```python
from build123d import *

# Parameters (mm, degrees)
SKETCH1_W                       = 1.5
SKETCH1_H                       = 25
BOSS_EXTRUDE1_DEPTH             = 73
BOSS_EXTRUDE1_DEPTH_BACK        = 73
FILLET1_R                       = 1
BOSS_EXTRUDE2_REACH             = 2.75
SKETCH10_W                      = 20
SKETCH10_H                      = 25
BOSS_EXTRUDE2_DIRECTION_2_REACH = 2.75
SKETCH16_W                      = 40.5
SKETCH16_H                      = 3
CUT_EXTRUDE2_DEPTH              = 10
SKETCH21_W                      = 65
SKETCH21_H                      = 47
BOSS_EXTRUDE4_DEPTH             = 1.5
FILLET4_R                       = 1.5
SKETCH17_W                      = 22.5
SKETCH17_H                      = 25
BOSS_EXTRUDE3_DEPTH             = 1.5
M2_CLEARANCE_HOLE4_D            = 2.4
M2_CLEARANCE_HOLE4_DEPTH        = 1.5
SKETCH22_OUTSIDE_W              = 183.058
SKETCH22_OUTSIDE_H              = 134.058
SKETCH22_OUTSIDE_W_2            = 125
SKETCH22_OUTSIDE_H_2            = 119
CUT_EXTRUDE4_DEPTH              = 10
M2_CLEARANCE_HOLE5_D            = 2.4
M2_CLEARANCE_HOLE5_DEPTH        = 11.5
SKETCH25_W                      = 65
SKETCH25_H                      = 2.5
SKETCH25_H_2                    = 0.5
BOSS_EXTRUDE5_DEPTH             = 1.5
M2_5_CLEARANCE_HOLE1_D          = 2.9
M2_5_CLEARANCE_HOLE1_DEPTH      = 11.5
SKETCH29_W                      = 7.5
SKETCH29_H                      = 30.5
SKETCH29_H_2                    = 50.5
CUT_EXTRUDE5_DEPTH              = 10
SKETCH31_W                      = 15
SKETCH31_H                      = 20.5
SKETCH31_H_2                    = 40.5
CUT_EXTRUDE7_DEPTH              = 10
FILLET5_R                       = 3
CHAMFER1_SIZE                   = 1.2
CHAMFER2_SIZE                   = 3
M2_5_CLEARANCE_HOLE2_D          = 2.9
M2_5_CLEARANCE_HOLE2_DEPTH      = 10


with BuildPart() as part:
    # Sketch1 → Boss-Extrude1 (new body, two sides)
    with BuildSketch(Plane.XY) as boss_extrude1_sk:
        Rectangle(SKETCH1_W, SKETCH1_H)
    extrude(amount=BOSS_EXTRUDE1_DEPTH)
    extrude(boss_extrude1_sk.sketch, amount=-BOSS_EXTRUDE1_DEPTH_BACK)

    # Fillet1
    fillet1_edges = [part.edges().sort_by_distance(p)[0] for p in [
        (0, -12.5, 73),
        (0, 12.5, -73),
        (0, 12.5, 73),
        (0, -12.5, -73),
    ]]
    fillet(fillet1_edges, radius=FILLET1_R)

    # Boss-Extrude2: up to this face of the body (flat: up to its plane)
    boss_extrude2_end = Plane(part.part.faces().sort_by_distance((0.75, 0, 0))[0])
    # Sketch10 → Boss-Extrude2 (add, up to the picked face)
    with BuildSketch(Plane(origin=(0, 0, 0), x_dir=(0, 0, -1), z_dir=(1, 0, 0)), mode=Mode.PRIVATE) as boss_extrude2_sk1:
        with Locations((0, 25)):
            Rectangle(SKETCH10_W, SKETCH10_H)
    boss_extrude2_tool1 = split(extrude(boss_extrude2_sk1.sketch, amount=BOSS_EXTRUDE2_REACH, mode=Mode.PRIVATE), bisect_by=boss_extrude2_end, keep=Keep.BOTH, mode=Mode.PRIVATE)
    add(boss_extrude2_tool1.solids().sort_by_distance((0, 25, 0))[0])

    # Boss-Extrude2 direction 2: up to this face of the body (flat: up to its plane)
    boss_extrude2_direction_2_end = Plane(part.part.faces().sort_by_distance((-0.75, 0, 0))[0])
    # Sketch10 → Boss-Extrude2 direction 2 (add, up to the picked face)
    with BuildSketch(Plane(origin=(0, 0, 0), x_dir=(0, 0, -1), z_dir=(1, 0, 0)), mode=Mode.PRIVATE) as boss_extrude2_direction_2_sk1:
        with Locations((0, 25)):
            Rectangle(SKETCH10_W, SKETCH10_H)
    boss_extrude2_direction_2_tool1 = split(extrude(boss_extrude2_direction_2_sk1.sketch, amount=-BOSS_EXTRUDE2_DIRECTION_2_REACH, mode=Mode.PRIVATE), bisect_by=boss_extrude2_direction_2_end, keep=Keep.BOTH, mode=Mode.PRIVATE)
    add(boss_extrude2_direction_2_tool1.solids().sort_by_distance((0, 25, 0))[0])

    # Sketch16 → Cut-Extrude2 (cut)
    with BuildSketch(Plane.ZY.offset(0.75)):
        with Locations((-52.75, 11)):
            Rectangle(SKETCH16_W, SKETCH16_H)
        with Locations((-52.75, -11)):
            Rectangle(SKETCH16_W, SKETCH16_H)
    cut_extrude2 = extrude(amount=-CUT_EXTRUDE2_DEPTH, mode=Mode.SUBTRACT)

    # Mirror3: Cut-Extrude2 across plane
    add(cut_extrude2.mirror(Plane.XY), mode=Mode.SUBTRACT)

    # Sketch21 → Boss-Extrude4 (add)
    with BuildSketch(Plane(origin=(0.75, 0, 0), x_dir=(0, 0, -1), z_dir=(1, 0, 0))):
        with Locations((0, -36)):
            Rectangle(SKETCH21_W, SKETCH21_H)
    extrude(amount=-BOSS_EXTRUDE4_DEPTH)

    # Fillet4
    fillet4_edges = [part.edges().sort_by_distance(p)[0] for p in [
        (0, 9.5, 73),
        (0, -9.5, 73),
        (0, 9.5, -73),
        (0, -9.5, -73),
    ]]
    fillet(fillet4_edges, radius=FILLET4_R)

    # Sketch17 → Boss-Extrude3 (add)
    with BuildSketch(Plane.ZY.offset(0.75)):
        with Locations((-21.25, 25)):
            Rectangle(SKETCH17_W, SKETCH17_H)
        with Locations((21.25, 25)):
            Rectangle(SKETCH17_W, SKETCH17_H)
    extrude(amount=-BOSS_EXTRUDE3_DEPTH)

    # M2 Clearance Hole4
    with Locations(Plane(origin=(0.75, 0, 0), x_dir=(0, 0, -1), z_dir=(1, 0, 0))):
        with Locations((20, 35), (-20, 35), (-20, -56), (20, -56)):
            Hole(M2_CLEARANCE_HOLE4_D / 2, depth=M2_CLEARANCE_HOLE4_DEPTH)

    # Sketch22 outside → Cut-Extrude4 (cut)
    with BuildSketch(Plane.ZY.offset(0.75)):
        with Locations((0, -11)):
            Rectangle(SKETCH22_OUTSIDE_W, SKETCH22_OUTSIDE_H)
        Rectangle(SKETCH22_OUTSIDE_W_2, SKETCH22_OUTSIDE_H_2, mode=Mode.SUBTRACT)
    extrude(amount=-CUT_EXTRUDE4_DEPTH, mode=Mode.SUBTRACT)

    # M2 Clearance Hole5
    with Locations(Plane(origin=(0.75, 0, 0), x_dir=(0, 0, -1), z_dir=(1, 0, 0))):
        with Locations((-54.5, -6.5), (-54.5, 6.5), (-59.5, 6.5), (-59.5, -6.5)):
            m2_clearance_hole5 = Hole(M2_CLEARANCE_HOLE5_D / 2, depth=M2_CLEARANCE_HOLE5_DEPTH)

    # Mirror4: M2 Clearance Hole5 across plane
    add(m2_clearance_hole5.mirror(Plane.XY), mode=Mode.SUBTRACT)

    # Sketch25 → Boss-Extrude5 (add)
    with BuildSketch(Plane(origin=(0.75, 0, 0), x_dir=(0, 0, -1), z_dir=(1, 0, 0))):
        with Locations((0, 38.75)):
            Rectangle(SKETCH25_W, SKETCH25_H)
        with Locations((0, -59.75)):
            Rectangle(SKETCH25_W, SKETCH25_H_2)
    extrude(amount=-BOSS_EXTRUDE5_DEPTH)

    # M2.5 Clearance Hole1
    with Locations(Plane(origin=(0.75, 0, 0), x_dir=(0, 0, -1), z_dir=(1, 0, 0))):
        with Locations((-5, -28), (5, -28), (5, 28), (-5, 28)):
            Hole(M2_5_CLEARANCE_HOLE1_D / 2, depth=M2_5_CLEARANCE_HOLE1_DEPTH)

    # Sketch29 → Cut-Extrude5 (cut)
    with BuildSketch(Plane(origin=(0.75, 0, 0), x_dir=(0, 0, -1), z_dir=(1, 0, 0))):
        with Locations((-28.75, 24.75)):
            Rectangle(SKETCH29_W, SKETCH29_H)
        with Locations((-28.75, -34.75)):
            Rectangle(SKETCH29_W, SKETCH29_H_2)
        with Locations((28.75, -34.75)):
            Rectangle(SKETCH29_W, SKETCH29_H_2)
        with Locations((28.75, 24.75)):
            Rectangle(SKETCH29_W, SKETCH29_H)
    extrude(amount=-CUT_EXTRUDE5_DEPTH, mode=Mode.SUBTRACT)

    # Sketch31 → Cut-Extrude7 (cut)
    with BuildSketch(Plane(origin=(0.75, 0, 0), x_dir=(0, 0, -1), z_dir=(1, 0, 0))):
        with Locations((-17.5, 19.75)):
            Rectangle(SKETCH31_W, SKETCH31_H)
        with Locations((-17.5, -29.75)):
            Rectangle(SKETCH31_W, SKETCH31_H_2)
        with Locations((17.5, -29.75)):
            Rectangle(SKETCH31_W, SKETCH31_H_2)
        with Locations((17.5, 19.75)):
            Rectangle(SKETCH31_W, SKETCH31_H)
    extrude(amount=-CUT_EXTRUDE7_DEPTH, mode=Mode.SUBTRACT)

    # Fillet5
    fillet5_edges = [part.edges().sort_by_distance(p)[0] for p in [
        (0, 30, 10),
        (0, 9.5, 10),
        (0, -9.5, 10),
        (0, -50, 10),
        (0, -9.5, -10),
        (0, -50, -10),
        (0, 9.5, -10),
        (0, 30, -10),
    ]]
    fillet(fillet5_edges, radius=FILLET5_R)

    # Chamfer1
    chamfer1_edges = [part.edges().sort_by_distance(p)[0] for p in [
        (0.75, -56, -21.2),
        (0.75, -56, 18.8),
        (0.75, 35, 18.8),
        (0.75, 35, -21.2),
        (0.75, -6.5, 58.3),
        (0.75, 6.5, 58.3),
        (0.75, 6.5, 53.3),
        (0.75, -6.5, 53.3),
    ]]
    chamfer(chamfer1_edges, length=CHAMFER1_SIZE)

    # Chamfer2
    chamfer2_edges = [part.edges().sort_by_distance(p)[0] for p in [
        (0, 40, 25),
        (0, -60, 25),
        (0, -60, -25),
        (0, 40, -25),
    ]]
    chamfer(chamfer2_edges, length=CHAMFER2_SIZE)

    # M2.5 Clearance Hole2
    with Locations(Plane.ZY.offset(0.75)):
        with Locations((-5.075, -5), (4.925, -5), (-5.075, 5), (4.925, 5)):
            Hole(M2_5_CLEARANCE_HOLE2_D / 2, depth=M2_5_CLEARANCE_HOLE2_DEPTH)


solid = part.part
```
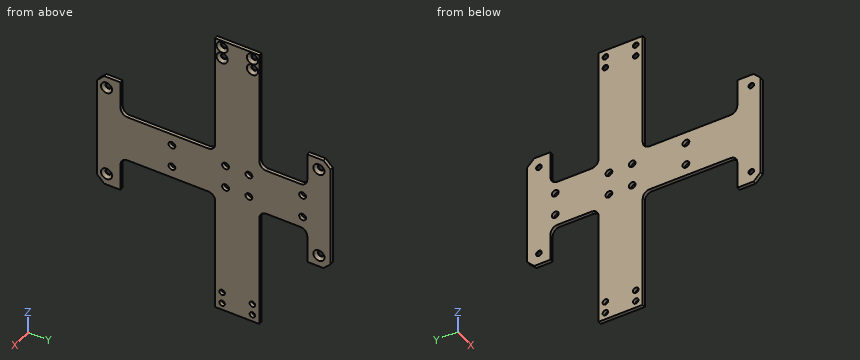
Work out the finished part from the listing and answer in its coordinate system (mm). Give positions to 0.01 mm unless a question says otherwise; leave off trailing zeros. Order: outer loops, then holes, each group sorted by start corner. A loop starts at its lowest first (then second) coordinate and runs counter-clockwise, first axis right, second up. Notation, with made-up numbers: (-18, 6) -> (-2, 6) arc R17 ccw to (-2, 12) -> close; hole circle Ø3 at (74, -25.5). An arc over 180 degrees is marked (long way). Answer as CSV lines item,"result". Start each with the question number.
(1) Section D-D, the plane z = 48 is taken. Write down the section's boundary in (x, y), plus the area to 3 significant figures.
(2) Section B-B, the plane z = -5 is taken. Write down the section's boundary in (x, y), plus the area to 3 significant figures.
(3) Consider line 1 along Y through (x, z) = (0.2, -5); line 2 along Y through (x, z) = (-0.55, -20); line 3 along Z through (x, y) = (-0.05, -4) (3 decimals). Determine where each line is inside the solid, lowest interval first.
(4) Each of these flat-tipped pins is pushed along its axis until it touches: pin 1 Ø4 at (y, z) = (-56, 20) entering from +X; pin 2 Ø0.8 at (x, y) = (0, 35) entering from +Z; pin 3 Ø0.8 at (x, y) = (-0.5, 33) entering from -Z. Where does it stop, or does it pass through?
(5) Section A-A, the plane y = -28 is taken. Write down the section's boundary in (x, z), plus the area to 3 significant figures.
(6) Section C-C, the plane x = 0.35 is taken. Give the number of separate pieces and of enclosed holes in the cut face, plus the area to 3 significant figures.
Entries:
1,outline,"(-0.75, -9.5) -> (0.75, -9.5) -> (0.75, 9.5) -> (-0.75, 9.5) -> close"
1,area,"28.5 mm²"
2,outline,"(-0.75, -60) -> (0.75, -60) -> (0.75, -29.45) -> (-0.75, -29.45) -> close; (-0.75, -26.55) -> (0.75, -26.55) -> (0.75, -6.45) -> (-0.75, -6.45) -> close; (-0.75, -3.55) -> (0.75, -3.55) -> (0.75, 3.55) -> (-0.75, 3.55) -> close; (-0.75, 6.45) -> (0.75, 6.45) -> (0.75, 26.55) -> (-0.75, 26.55) -> close; (-0.75, 29.45) -> (0.75, 29.45) -> (0.75, 40) -> (-0.75, 40) -> close"
2,area,"133 mm²"
3,line 1,"-60 to -29.45, -26.55 to -6.45, -3.55 to 3.55, 6.45 to 26.55, 29.45 to 40"
3,line 2,"-60 to -57.2, -54.8 to -50, -9.5 to 9.5, 30 to 33.8, 36.2 to 40"
3,line 3,"-62.5 to -6.125, -4.025 to 3.875, 5.975 to 62.5"
4,pin 1,"x = 0.35"
4,pin 2,"z = 25"
4,pin 3,"z = -25"
5,outline,"(-0.75, -10) -> (0.75, -10) -> (0.75, -6.45) -> (-0.75, -6.45) -> close; (-0.75, -3.55) -> (0.75, -3.55) -> (0.75, 3.55) -> (-0.75, 3.55) -> close; (-0.75, 6.45) -> (0.75, 6.45) -> (0.75, 10) -> (-0.75, 10) -> close"
5,area,"21.3 mm²"
6,separate pieces,"1"
6,enclosed holes,"20"
6,area,"4,420 mm²"
